For this review, take the finished solid that the model builds, in its own axes (mm). A direction names the side the tool comes from. Coordinates: 2 decimals unless noted, no trailing zeros. Write each loop counter-clockwise with the first axis right and the second up, starting at its lowest first coordinate (ties: lowest second). Pieces come first, ordered by that corner, then holes.
```python
from build123d import *

# Parameters (mm, degrees)
BASE_FLANGE1_DEPTH = 362
SKETCH6_R          = 4
CUT_EXTRUDE1_DEPTH = 10


# Sheet-metal steps are written as plain solids
with BuildPart() as part:
    # Sketch1 → Base-Flange1 (new body)
    with BuildSketch(Plane.XY):
        with BuildLine():
            Line((0, 50), (0, 3))
            ThreePointArc((0, 3), (0.878679656, 0.878679656), (3, 0))
            Line((3, 0), (397, 0))
            ThreePointArc((397, 0), (399.121320344, 0.878679656), (400, 3))
            Line((400, 3), (400, 50))
            Line((400, 50), (398, 50))
            Line((398, 50), (398, 3))
            ThreePointArc((398, 3), (397.707106781, 2.292893219), (397, 2))
            Line((397, 2), (3, 2))
            ThreePointArc((3, 2), (2.292893219, 2.292893219), (2, 3))
            Line((2, 3), (2, 50))
            Line((2, 50), (0, 50))
        make_face()
    extrude(amount=BASE_FLANGE1_DEPTH)

    # Sketch6 → Cut-Extrude1 (cut)
    with BuildSketch(Plane.XZ):
        with Locations(Location((53, 322, 0), (0, 0, 270))):
            Circle(SKETCH6_R)
        with Locations(Location((83, 322, 0), (0, 0, 270))):
            Circle(SKETCH6_R)
        with Locations(Location((83, 282, 0), (0, 0, 270))):
            Circle(SKETCH6_R)
        with Locations(Location((53, 282, 0), (0, 0, 270))):
            Circle(SKETCH6_R)
        with Locations(Location((347, 282, 0), (0, 0, 270))):
            Circle(SKETCH6_R)
        with Locations(Location((317, 282, 0), (0, 0, 270))):
            Circle(SKETCH6_R)
        with Locations(Location((317, 322, 0), (0, 0, 270))):
            Circle(SKETCH6_R)
        with Locations(Location((347, 322, 0), (0, 0, 270))):
            Circle(SKETCH6_R)
    extrude(amount=-CUT_EXTRUDE1_DEPTH, mode=Mode.SUBTRACT)


solid = part.part
```
1) Tool access review of faces 4 (the face through (398, 27, 178)), 5 (the face through (400, 26, 178)): name each direction out of +Z, -Z, +X, -X, +Y, -Y from which nothing blocks a thin tool from reaching the whole face with its end or side.
2) For L1, parallel to Z at x = 317, y = 0.75; L2, parallel to X at y = 22, z = 111.5; L3, parallel to X at y = 1.35, z = 282, list the stretches that pass through material, from the lowest coordinate up.
3) Clearance check with flat-ended pins moving along their axes: P1, Ø8, axis at y = 12.5, z = 231.5, coming from the -X side; P2, Ø6.5, axis at x = 53, z = 322, coming from the +Y side; P3, Ø1.5, axis at x = 340, z = 241, coming from the +Y side. State where each tip first meets the part, or that it passes through.
4) Consider section A-A (y = 36.5). Give the boundary of the cut face in (x, z), then the cut area to 3 significant figures.
5) Consider section B-B (z = 48). Give the boundary of the cut face in (x, y).
6) Consider section C-C (x = 231). Give the boundary of the cut face in (y, z), then the cut area to 3 significant figures.
7) The part is to be moulded in two halves that separate along X. For faces 1 (the face through (197, 0, 178)), 2 (the face through (0, 27, 178)), 3 (the face through (2, 26, 178)), say which applies: pulls with the +X half, pulls with the -X half, needs draft (parallel to the pull), parting line crosses it, or undercut.
Results:
1. face 4: +Z, -Z, +Y
1. face 5: +Z, -Z, +X, +Y, -Y
2. L1: z = 0 to 278, 286 to 318, 326 to 362
2. L2: x = 0 to 2, 398 to 400
2. L3: x = 0.49 to 49, 57 to 79, 87 to 313, 321 to 343, 351 to 399.51
3. P1: stops at x = 0
3. P2: passes through
3. P3: stops at y = 2
4. outline: (0, 0) - (2, 0) - (2, 362) - (0, 362) - close; (398, 0) - (400, 0) - (400, 362) - (398, 362) - close
4. area: 1,450 mm2
5. outline: (0, 3) arc R3 ccw to (3, 0) - (397, 0) arc R3 ccw to (400, 3) - (400, 50) - (398, 50) - (398, 3) arc R1 cw to (397, 2) - (3, 2) arc R1 cw to (2, 3) - (2, 50) - (0, 50) - close
6. outline: (0, 0) - (2, 0) - (2, 362) - (0, 362) - close
6. area: 724 mm2
7. face 1: needs draft
7. face 2: pulls with the -X half
7. face 3: undercut
